Part model, mm, in its own coordinate system. A direction names the side the tool comes from. Round coordinates to 2 decimals unless told otherwise and drop trailing zeros. Loops run counter-clockwise (first coordinate to the right, second up) from the corner with the lowest first, then second, coordinate; pieces in that order, holes last. Notation, with made-up numbers: M 22,-39.75 L 62,-39.75 A15 ccw 62,-15.75 Z; hole C 27.25,39.25 d4. An arc over 180 degrees is marked long. Answer as CSV lines item,"result". Start each with the question number.
Item 1: Band-saw the part on C-C (z = 3.75). Give the cut face in (x, y) (3 decimals), and give its area (3 significant figures).
Item 2: Band-saw the part on D-D (y = -37). Give the cut face in (x, z) (3 decimals).
Item 3: Wall check: line 1 (Y direction, x = 39, z = 5.25) (3 decimals); line 2 (X direction, y = 29, z = 5.75) (3 decimals); line 3 (X direction, y = 34.5, z = 0.75) (3 decimals). Give the ranges that are in metal, low to high.
Item 4: Which spindle directions (+Z, -Z, +X, -X, +Y, -Y) get a long thin tool onto all of the face, cutting with end or side? Do faces 1 (the flat face through (-3.175, 3, 3)), 2 (the conical face through (-52.45, 52.7, 2.01)). Say none if no direction does.
Item 5: Drop flat-ended pins along their axis: pin 1 Ø1 at (x, z) = (45, 3) entering from +Y; pin 2 Ø7.5 at (x, y) = (41.275, 31.75) entering from +Z; pin 3 Ø1.5 at (x, z) = (19.5, 0.5) entering from -Y; pin 4 Ø1.9 at (y, z) = (9.5, 2.5) entering from +X. Give the stop position or say it passes through.
Item 6: Mould opens along Y. For faces 3 (the cylindrical face through (40.59, 28.65, 3.13)), 4 (the flat face through (35.014, 57.821, 2.576)), 5 (the flat face through (-57.821, 35.014, 2.576)) say: pulls with the +Y half, pulls with the -Y half, needs draft (parallel to the pull), parting line crosses it, or undercut.
Item 7: Band-saw the part on B-B (x = 0). Give the cut face in (y, z).
Item 8: Band-saw the part on A-A (y = 31.75). Give the cut face in (x, z) (3 decimals), and give its area (3 significant figures).
```python
from build123d import *

# Parameters (mm, degrees)
F0_W     = 120.65
F0_H     = 120.65
F0_R     = 3.175
F1_DEPTH = 6.35
F4_DEPTH = 25.4
F5_R     = 3.175
F6_DEPTH = 25.4
F7_SIZE  = 5.08


# Not quite as in the source:
# - a feature of the source that left no trace in its solid (it failed there, or was rolled back) is left out


with BuildPart() as f1:
    # F0 (on Top) → F1 (new body)
    with BuildSketch(Plane.XY):
        Rectangle(F0_W, F0_H)
        with Locations((-41.275, -31.75)):
            Circle(F0_R, mode=Mode.SUBTRACT)
        with Locations((41.275, -31.75)):
            Circle(F0_R, mode=Mode.SUBTRACT)
        with Locations((-41.275, 31.75)):
            Circle(F0_R, mode=Mode.SUBTRACT)
        with Locations((41.275, 31.75)):
            Circle(F0_R, mode=Mode.SUBTRACT)
    extrude(amount=F1_DEPTH)

    # F2 (on face) → F4 (cut)
    with BuildSketch(Plane(origin=(0, 0, 0), x_dir=(1, 0, 0), z_dir=(0, 0, -1))):
        with BuildLine():
            ThreePointArc((-3.175, -15.875), (0, -19.05), (3.175, -15.875))
            ThreePointArc((3.175, -15.875), (0, -12.7), (-3.175, -15.875))
        make_face()
        with BuildLine():
            ThreePointArc((-3.175, -15.875), (0, -12.7), (3.175, -15.875))
            Line((3.1750000339, -15.875), (3.1713092382, 9.3719551838))
            ThreePointArc((3.1713092382, 9.3719551838), (-0.0765446561, 6.3509228246), (-3.175, 9.525))
            Line((-3.175, 9.525), (-3.175, -15.875))
        make_face()
        with BuildLine():
            Line((3.1712643561, 9.6789720229), (3.1713092382, 9.3719551838))
            ThreePointArc((3.1713092382, 9.3719551838), (3.1740771754, 9.4484553439), (3.175, 9.525))
            ThreePointArc((3.175, 9.525), (3.1740659516, 9.6020086665), (3.1712643561, 9.6789720229))
        make_face()
        with BuildLine():
            ThreePointArc((-3.175, 9.525), (-0.0765446561, 6.3509228246), (3.1713092382, 9.3719551838))
            Line((3.1713092382, 9.3719551838), (3.1712643561, 9.6789720229))
            ThreePointArc((3.1712643561, 9.6789720229), (-0.0770086665, 12.6990659516), (-3.175, 9.525))
        make_face()
    extrude(amount=-F4_DEPTH, mode=Mode.SUBTRACT)

    # F5 (on face) → F6 (cut)
    with BuildSketch(Plane.XY.offset(6.35)):
        with BuildLine():
            ThreePointArc((-28.575, 60.325), (0, 54.7642905896), (28.575, 60.325))
            Line((28.575, 60.325), (-28.575, 60.325))
        make_face()
        with BuildLine():
            Line((-28.575, -60.325), (28.575, -60.325))
            ThreePointArc((28.575, -60.325), (0, -54.7642905896), (-28.575, -60.325))
        make_face()
        with BuildLine():
            Line((60.325, -28.575), (60.325, 28.575))
            ThreePointArc((60.325, 28.575), (54.7642905896, 0), (60.325, -28.575))
        make_face()
        with BuildLine():
            ThreePointArc((-60.325, -28.575), (-54.7642905896, 0), (-60.325, 28.575))
            Line((-60.325, 28.575), (-60.325, -28.575))
        make_face()
        with Locations((41.275, 31.75)):
            Circle(F5_R)
        with Locations((41.275, -31.75)):
            Circle(F5_R)
        with Locations((-41.275, -31.75)):
            Circle(F5_R)
        with Locations((-41.275, 31.75)):
            Circle(F5_R)
        with BuildLine():
            Line((60.325, 60.325), (41.275, 60.325))
            ThreePointArc((41.275, 60.325), (54.7453841816, 54.7453841816), (60.325, 41.275))
            Line((60.325, 41.275), (60.325, 60.325))
        make_face()
        with BuildLine():
            ThreePointArc((-41.275, -60.325), (-54.7453841816, -54.7453841816), (-60.325, -41.275))
            Line((-60.325, -41.275), (-60.325, -60.325))
            Line((-60.325, -60.325), (-41.275, -60.325))
        make_face()
        with BuildLine():
            ThreePointArc((-60.325, 41.275), (-54.7453841816, 54.7453841816), (-41.275, 60.325))
            Line((-41.275, 60.325), (-60.325, 60.325))
            Line((-60.325, 60.325), (-60.325, 41.275))
        make_face()
        with BuildLine():
            Line((60.325, -60.325), (60.325, -41.275))
            ThreePointArc((60.325, -41.275), (54.7453841816, -54.7453841816), (41.275, -60.325))
            Line((41.275, -60.325), (60.325, -60.325))
        make_face()
    extrude(amount=-F6_DEPTH, mode=Mode.SUBTRACT)

    # F7
    f7_edges = [f1.edges().sort_by_distance(p)[0] for p in [
        (0, 54.764291, 0),
        (54.745384, 54.745384, 0),
        (54.764291, 0, 0),
        (54.745384, -54.745384, 0),
        (-34.925, -60.325, 0),
        (0, -54.764291, 0),
        (-54.745384, 54.745384, 0),
        (-60.325, 34.925, 0),
        (-54.764291, 0, 0),
        (-54.745384, -54.745384, 0),
        (-60.325, -34.925, 0),
        (-34.925, 60.325, 0),
        (34.925, 60.325, 0),
        (60.325, 34.925, 0),
        (60.325, -34.925, 0),
        (34.925, -60.325, 0),
    ]]
    chamfer(f7_edges, length=F7_SIZE)


solid = f1.part
```
Answer block:
1,outline,"M -58.995,-41.275 A17.72 ccw -41.275,-58.995 L -28.833,-58.995 A77.53 cw 28.833,-58.995 L 41.275,-58.995 A17.72 ccw 58.995,-41.275 L 58.995,-28.833 A77.53 cw 58.995,28.833 L 58.995,41.275 A17.72 ccw 41.275,58.995 L 28.833,58.995 A77.53 cw -28.833,58.995 L -41.275,58.995 A17.72 ccw -58.995,41.275 L -58.995,28.833 A77.53 cw -58.995,-28.833 Z; hole C -41.275,-31.75 d6.35; hole C -41.275,31.75 d6.35; hole M -3.175,-9.525 A3.175 ccw long 3.171,-9.372 L 3.175,15.875 A3.175 ccw -3.175,15.875 Z; hole C 41.275,-31.75 d6.35; hole C 41.275,31.75 d6.35"
1,area,"12,500 mm^2"
2,outline,"M -60.325,5.08 L -55.245,0 L 55.245,0 L 60.325,5.08 L 60.325,6.35 L -60.325,6.35 Z"
3,line 1,"y = -60.325 to -33.965, -29.535 to 29.535, 33.965 to 60.325"
3,line 2,"x = -60.325 to -42.862, -39.688 to 39.688, 42.862 to 60.325"
3,line 3,"x = -55.995 to -42.862, -39.688 to 39.688, 42.862 to 55.995"
4,face 1,"+Z, -Z"
4,face 2,"-Z, -X, +Y"
5,pin 1,"stops at y = 58.35"
5,pin 2,"stops at z = 6.35"
5,pin 3,"stops at y = -53.37"
5,pin 4,"stops at x = 53.72"
6,face 3,"undercut"
6,face 4,"pulls with the +Y half"
6,face 5,"needs draft"
7,outline,"M -54.76,5.08 L -49.68,0 L -12.7,0 L -12.7,6.35 L -54.76,6.35 Z; M 19.05,0 L 49.68,0 L 54.76,5.08 L 54.76,6.35 L 19.05,6.35 Z"
8,outline,"M -60.325,5.08 L -55.245,0 L -44.45,0 L -44.45,6.35 L -60.325,6.35 Z; M -38.1,0 L 38.1,0 L 38.1,6.35 L -38.1,6.35 Z; M 44.45,0 L 55.245,0 L 60.325,5.08 L 60.325,6.35 L 44.45,6.35 Z"
8,area,"660 mm^2"
